Read the model definition and answer for the solid it produces. Units are mm, in the model's axes. A direction names the side the tool comes from. Give positions to 0.01 mm unless a question says otherwise; leave off trailing zeros. Loops run counter-clockwise (first coordinate to the right, second up) from the corner with the lowest first, then second, coordinate; pieces in that order, holes last. Notation, with made-up numbers: (-15, 12) - (32, 12) arc R12 ccw to (32, 35) - close; hole circle Ø1 at (4.5, -13.75). An arc over 180 degrees is marked (long way). Use a Markdown table: item, result. Add a question column.
Item 1: For a pull along Z with two mould halves and no side action, classify faces 4 (the face through (-654.23, 47, 219)), 5 (the face through (-803.41, 64.61, 371.7)), 6 (the face through (-712, 22, 0)), 7 (the face through (-657, 44, 444.5)) as +Z half, -Z half, draft (parallel to the pull), parting line (faces both ways), or undercut.
Item 2: A cutting plane is placed at A-A (z = 42). Determine the outline of the cut face in (x, y), plus the area to 3 significant figures.
Item 3: Each of these flat-tipped pins is pushed along its axis until it touches: P1, Ø1.9, axis at x = -713.5, y = 33, coming from the +Z side; P2, Ø12, axis at x = -683.5, z = 178, coming from the +Y side; P3, Ø1.9, axis at x = -644, y = -4.5, coming from the +Z side. Where does it stop, or does it pass through?
Item 4: A cutting plane is placed at B-B (y = 82). Determine the outline of the cut face in (x, z), plus the area to 3 significant figures.
Item 5: Which of the six approach directions +Z, -Z, +X, -X, +Y, -Y give full straight-line access (tool end or side, diameter ignored) to faces 1 (the face through (-717.73, 47, 194)), 2 (the face through (-582, 0, 225)), 3 (the face through (-806.63, 44, 219))?
Item 6: A cutting plane is placed at D-D (y = 29.5). Determine the outline of the cut face in (x, z).
Item 7: Consider probe 1 along X at (y, z) = (7, 66); probe 2 along X at (y, z) = (1.5, 395); probe 3 along X at (y, z) = (19.5, 38). Determine where each line is inside the solid, lowest interval first. Write a range as [from, to].
Item 8: A cutting plane is placed at C-C (z = 381). Determine the outline of the cut face in (x, y), plus the area to 3 significant figures.
from build123d import *

# Parameters (mm, degrees)
F0_W      = 298.45
F0_H      = 444.5
F1_DEPTH  = 6.35
F2_W      = 6.35
F2_H      = 444.5
F3_DEPTH  = 95.25
F4_W      = 6.35
F4_H      = 57.15
F5_DEPTH  = 6.351
F6_W      = 6.35
F6_H      = 444.5
F7_DEPTH  = 95.25
F8_W      = 19.05
F8_H      = 50.8
F9_W      = 95.25
F9_H      = 50.8
F10_DEPTH = 25.4
F11_W     = 139.7
F11_H     = 12.7
F12_DEPTH = 25.4
F13_R     = 9.525
F14_DEPTH = 25.4


with BuildPart() as f1:
    # F0 (on Front) → F1 (new body)
    with BuildSketch(Plane.XZ):
        with Locations((-657.405383, 222.25)):
            Rectangle(F0_W, F0_H)
    extrude(amount=F1_DEPTH)

    # F2 (on face) → F3 (join)
    with BuildSketch(Plane(origin=(0, 0, 0), x_dir=(-1, 0, 0), z_dir=(0, 1, 0))):
        with Locations((803.455383, 222.25)):
            Rectangle(F2_W, F2_H)
    extrude(amount=F3_DEPTH)

    # F4 (on face) → F5 (cut, through all)
    with BuildSketch(Plane(origin=(0, 0, 0), x_dir=(-1, 0, 0), z_dir=(0, 1, 0))):
        with Locations((517.705383, 415.925)):
            Rectangle(F4_W, F4_H)
        with Locations((530.405383, 415.925)):
            Rectangle(F4_W, F4_H)
        with Locations((543.105383, 415.925)):
            Rectangle(F4_W, F4_H)
        with Locations((555.805383, 415.925)):
            Rectangle(F4_W, F4_H)
        with Locations((568.505383, 415.925)):
            Rectangle(F4_W, F4_H)
        with Locations((581.205383, 415.925)):
            Rectangle(F4_W, F4_H)
        with Locations((593.905383, 415.925)):
            Rectangle(F4_W, F4_H)
        with Locations((606.605383, 415.925)):
            Rectangle(F4_W, F4_H)
        with Locations((619.305383, 415.925)):
            Rectangle(F4_W, F4_H)
        with Locations((632.005383, 415.925)):
            Rectangle(F4_W, F4_H)
        with Locations((644.705383, 415.925)):
            Rectangle(F4_W, F4_H)
    extrude(amount=-F5_DEPTH, mode=Mode.SUBTRACT)

    # F6 (on face) → F7 (join)
    with BuildSketch(Plane(origin=(0, 0, 0), x_dir=(-1, 0, 0), z_dir=(0, 1, 0))):
        with Locations((657.405383, 222.25)):
            Rectangle(F6_W, F6_H)
        with Locations((714.555383, 222.25)):
            Rectangle(F6_W, F6_H)
    extrude(amount=F7_DEPTH)

    # F8 (on face) + F9 (on face) → F10 (cut)
    with BuildSketch(Plane.YZ.offset(-654.230383)):
        with Locations((28.575, 25.4)):
            Rectangle(F8_W, F8_H)
        with Locations((66.675, 25.4)):
            Rectangle(F8_W, F8_H)
    with BuildSketch(Plane.YZ.offset(-711.380383)):
        with Locations((47.625, 419.1)):
            Rectangle(F9_W, F9_H)
    extrude(amount=-F10_DEPTH, mode=Mode.SUBTRACT)

    # F11 (on face) → F12 (cut)
    with BuildSketch(Plane(origin=(0, 0, 0), x_dir=(-1, 0, 0), z_dir=(0, 1, 0))):
        with Locations((730.430383, 438.15)):
            Rectangle(F11_W, F11_H)
    extrude(amount=-F12_DEPTH, mode=Mode.SUBTRACT)

    # F13 (on face) → F14 (cut)
    with BuildSketch(Plane.YZ.offset(-800.280383)):
        with Locations((66.675, 381)):
            Circle(F13_R)
    extrude(amount=-F14_DEPTH, mode=Mode.SUBTRACT)


solid = f1.part
Geometry says:
| question | item | result |
|---|---|---|
| 1 | face 4 | draft |
| 1 | face 5 | undercut |
| 1 | face 6 | -Z half |
| 1 | face 7 | +Z half |
| 2 | outline | (-806.63, -6.35) - (-508.18, -6.35) - (-508.18, 0) - (-654.23, 0) - (-654.23, 19.05) - (-660.58, 19.05) - (-660.58, 0) - (-711.38, 0) - (-711.38, 95.25) - (-717.73, 95.25) - (-717.73, 0) - (-800.28, 0) - (-800.28, 95.25) - (-806.63, 95.25) - close; (-660.58, 38.1) - (-654.23, 38.1) - (-654.23, 57.15) - (-660.58, 57.15) - close; (-660.58, 76.2) - (-654.23, 76.2) - (-654.23, 95.25) - (-660.58, 95.25) - close |
| 2 | area | 3,470 mm² |
| 3 | P1 | z = 393.7 |
| 3 | P2 | y = 0 |
| 3 | P3 | z = 387.35 |
| 4 | outline | (-806.63, 0) - (-800.28, 0) - (-800.28, 444.5) - (-806.63, 444.5) - close; (-717.73, 0) - (-711.38, 0) - (-711.38, 393.7) - (-717.73, 393.7) - close; (-660.58, 0) - (-654.23, 0) - (-654.23, 444.5) - (-660.58, 444.5) - close |
| 4 | area | 8,150 mm² |
| 5 | face 1 | +Z, -Z, +Y |
| 5 | face 2 | +Z, -Z, +X, +Y |
| 5 | face 3 | +Z, -Z, -X, +Y, -Y |
| 6 | outline | (-806.63, 0) - (-800.28, 0) - (-800.28, 444.5) - (-806.63, 444.5) - close; (-717.73, 0) - (-711.38, 0) - (-711.38, 393.7) - (-717.73, 393.7) - close; (-660.58, 50.8) - (-654.23, 50.8) - (-654.23, 444.5) - (-660.58, 444.5) - close |
| 7 | probe 1 | [-806.63, -800.28], [-717.73, -711.38], [-660.58, -654.23] |
| 7 | probe 2 | [-806.63, -800.28], [-660.58, -654.23] |
| 7 | probe 3 | [-806.63, -800.28], [-717.73, -711.38] |
| 8 | outline | (-806.63, -6.35) - (-508.18, -6.35) - (-508.18, 0) - (-654.23, 0) - (-654.23, 95.25) - (-660.58, 95.25) - (-660.58, 0) - (-711.38, 0) - (-711.38, 95.25) - (-717.73, 95.25) - (-717.73, 0) - (-800.28, 0) - (-800.28, 57.15) - (-806.63, 57.15) - close; (-806.63, 76.2) - (-800.28, 76.2) - (-800.28, 95.25) - (-806.63, 95.25) - close |
| 8 | area | 3,590 mm² |
